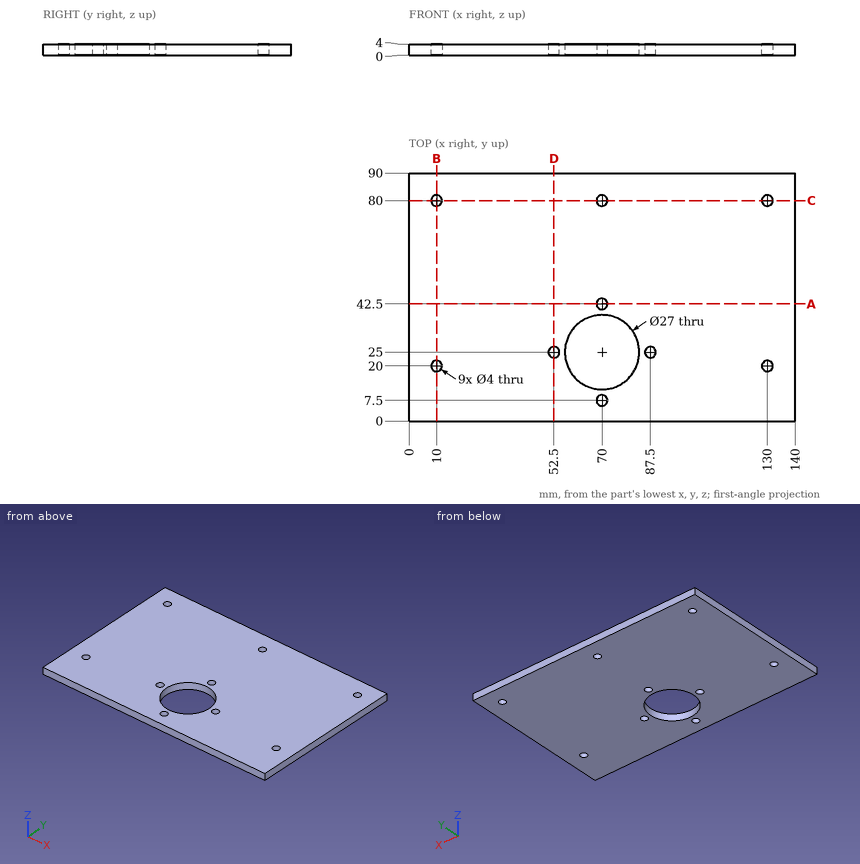
Design review of the part shown in the three views and the two pictorial views. Dimensions are in mm from the part's minimum x, y and z. Round coordinates to 2 decimals unless told otherwise and drop trailing zeros. Write each loop counter-clockwise with the first axis right and the second up, starting at its lowest first coordinate (ties: lowest second). Pieces come first, ordered by that corner, then holes. Notation, with made-up numbers: M 76.25,-3.75 L 131.25,-3.75 A19 ccw 131.25,0.25 Z; hole C 63.25,37.5 d6. An arc over 180 degrees is marked long. Use a Markdown table: item, result. Add a question column.
Q1. To check wall thickness, follow line 1 (Y direction, x = 10, z = 2.6); line 2 (X direction, y = 80, z = 1.15); line 3 (Y direction, x = 70, z = 2.65). State the ranges of each line that lie inside material, in increasing order.
Q2. We need section D-D, the plane x = 52.5. State the section outline as (y, z) points.
Q3. Insertion check: pin 1 (2.5 mm diameter, centred on x = 130, y = 80, fed in from -Z). The pin has a flat end and moves straight along its axis. Give the tip position at first contact, or say it passes through.
Q4. We need section A-A, the plane y = 42.5. State the section outline as (x, z) points.
Q5. We need section C-C, the plane y = 80. State the section outline as (x, z) points, plus the area to 3 significant figures.
Q6. We need section B-B, the plane x = 10. State the section outline as (y, z) points.
Findings below:
| question | item | result |
|---|---|---|
| 1 | line 1 | y = 0 to 18, 22 to 78, 82 to 90 |
| 1 | line 2 | x = 0 to 8, 12 to 68, 72 to 128, 132 to 140 |
| 1 | line 3 | y = 0 to 5.5, 9.5 to 11.5, 38.5 to 40.5, 44.5 to 78, 82 to 90 |
| 2 | outline | M 0,0 L 23,0 L 23,4 L 0,4 Z; M 27,0 L 90,0 L 90,4 L 27,4 Z |
| 3 | pin 1 | passes through |
| 4 | outline | M 0,0 L 68,0 L 68,4 L 0,4 Z; M 72,0 L 140,0 L 140,4 L 72,4 Z |
| 5 | outline | M 0,0 L 8,0 L 8,4 L 0,4 Z; M 12,0 L 68,0 L 68,4 L 12,4 Z; M 72,0 L 128,0 L 128,4 L 72,4 Z; M 132,0 L 140,0 L 140,4 L 132,4 Z |
| 5 | area | 512 mm² |
| 6 | outline | M 0,0 L 18,0 L 18,4 L 0,4 Z; M 22,0 L 78,0 L 78,4 L 22,4 Z; M 82,0 L 90,0 L 90,4 L 82,4 Z |
